from build123d import *

# Parameters (mm, degrees)
F0_R     = 4
F0_R_2   = 2.5
F1_DEPTH = 5
F2_START = 2
F2_DEPTH = 3
F3_DEPTH = 50
F4_SIZE  = 0.5


with BuildPart() as f1:
    # F0 (on Top) → F1 (new body)
    with BuildSketch(Plane.XY):
        Circle(F0_R)
        Circle(F0_R_2, mode=Mode.SUBTRACT)
        Circle(F0_R_2)
        Polygon((2.3094010768, 0), (1.1547005384, -2), (-1.1547005384, -2), (-2.3094010768, 0), (-1.1547005384, 2), (1.1547005384, 2), align=None, mode=Mode.SUBTRACT)
        Polygon((-1.1547005384, -2), (1.1547005384, -2), (2.3094010768, 0), (1.1547005384, 2), (-1.1547005384, 2), (-2.3094010768, 0), align=None)
    extrude(amount=F1_DEPTH)

    # F0 (on Top) → F2 (cut)
    with BuildSketch(Plane.XY.offset(F2_START)):
        Polygon((-1.1547005384, -2), (1.1547005384, -2), (2.3094010768, 0), (1.1547005384, 2), (-1.1547005384, 2), (-2.3094010768, 0), align=None)
    extrude(amount=F2_DEPTH, mode=Mode.SUBTRACT)

    # F0 (on Top) → F3 (join)
    with BuildSketch(Plane.XY):
        Circle(F0_R_2)
        Polygon((2.3094010768, 0), (1.1547005384, -2), (-1.1547005384, -2), (-2.3094010768, 0), (-1.1547005384, 2), (1.1547005384, 2), align=None, mode=Mode.SUBTRACT)
        Polygon((-1.1547005384, -2), (1.1547005384, -2), (2.3094010768, 0), (1.1547005384, 2), (-1.1547005384, 2), (-2.3094010768, 0), align=None)
    extrude(amount=-F3_DEPTH)

    # F4
    f4_edges = [f1.edges().sort_by_distance(p)[0] for p in [
        (-4, 0, 5),
    ]]
    chamfer(f4_edges, length=F4_SIZE)


solid = f1.part
Verification items for the finished model (mm, model axes). A direction names the side the tool comes from. Give positions to 0.01 mm unless a question says otherwise; leave off trailing zeros. Order: outer loops, then holes, each group sorted by start corner. A loop starts at its lowest first (then second) coordinate and runs counter-clockwise, first axis right, second up. Notation, with made-up numbers: M -26.5,-5.75 L -20.5,-5.75 A34 ccw -20.5,27.25 Z; hole C 37.25,35.25 d9. An arc over 180 degrees is marked long. Use one line per item in the form item = value. Start each with the question number.
Q1. Section check C-C (z = -47). Enter the section's corners in (x, y).
Q2. Access from +Z, -Z, +X, -X, +Y, -Y to the whole of each face (thin tool, end or side, straight path). Record for faces 1 (the flat face through (-1.724, 1.014, 3.479)), 2 (the cylindrical face through (-0.867, -3.905, 2.218)), 3 (the flat face through (2, 2, 0)).
Q3. Go/stop test with flat-tipped pins: pin 1 Ø1 at (y, z) = (-1, -17.5) entering from -X; pin 2 Ø2 at (y, z) = (1, -23) entering from -X; pin 3 Ø1 at (x, z) = (-2, -44) entering from -Y. Record where each tip stops, or that it passes through.
Q4. Section check B-B (z = 0.5). Enter the section's corners in (x, y), then the cut area to 3 significant figures.
Q5. Mould release check, pull along Y, two halves, no side actions. Record for faces 4 (the flat face through (0, 2, 3)), 5 (the flat face through (0, 0, 2)), 6 (the cylindrical face through (-0.54, -2.44, -24.65)), 7 (the flat face through (0, 0, -50)): +Y half, -Y half, draft (parallel to the pull), parting line (faces both ways), or undercut.
Q6. Section check A-A (x = 0). Enter the section's corners in (y, z), then the cut area to 3 significant figures.
Q7. Scan lines: line 1 along Y through (x, z) = (-1.5, -4.5); line 2 along Z through (x, y) = (1, 2.75). Record each from-to range of solid material in increasing order. Write a range as [from, to].
Evaluation:
q1.outline = C 0,0 d5
q2.face_1 = +Z
q2.face_2 = +Z, -Z
q2.face_3 = -Z
q3.pin_1 = -2.45
q3.pin_2 = -2.5
q3.pin_3 = -2
q4.outline = C 0,0 d8
q4.area = 50.3 mm2
q5.face_4 = undercut
q5.face_5 = undercut
q5.face_6 = parting line
q5.face_7 = draft
q6.outline = M -4,0 L -2.5,0 L -2.5,-50 L 2.5,-50 L 2.5,0 L 4,0 L 4,4.5 L 3.5,5 L 2,5 L 2,2 L -2,2 L -2,5 L -3.5,5 L -4,4.5 Z
q6.area = 278 mm2
q7.line_1 = [-2, 2]
q7.line_2 = [0, 5]
